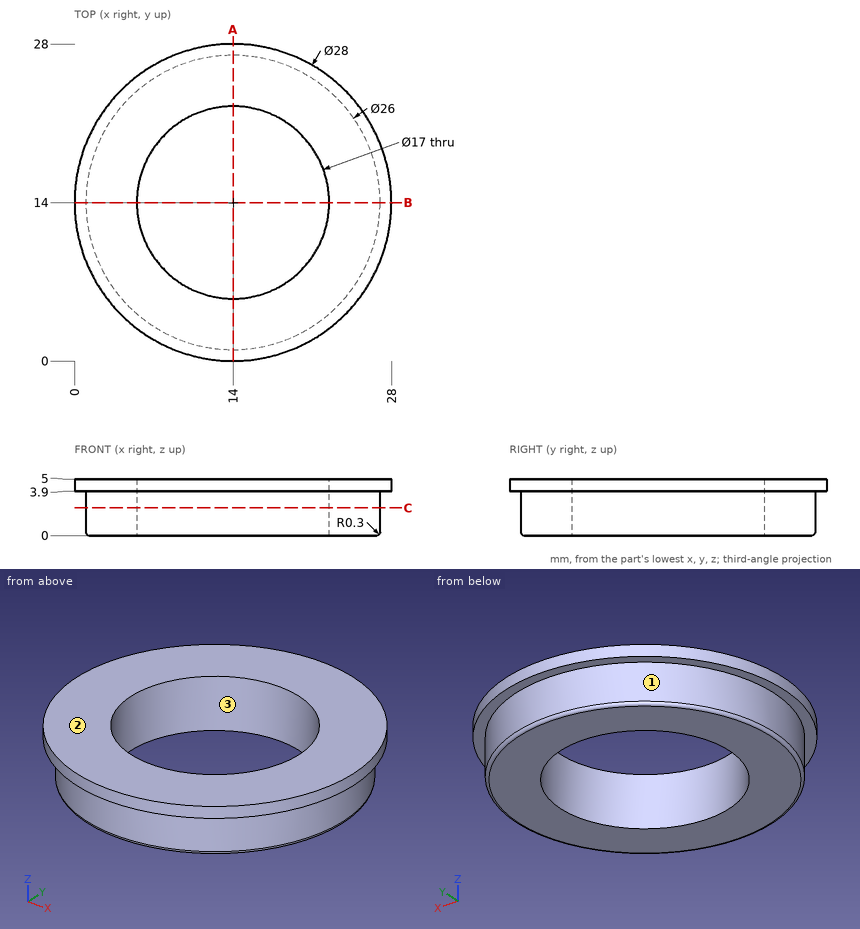
Study the drawing (mm; zero at the part's minimum x, y, z) and answer. Give positions to 0.01 mm unless a question says otherwise; leave off trailing zeros. Loops run counter-clockwise (first coordinate to the right, second up) from the corner with the lowest first, then second, coordinate; pieces in that order, holes last. Notation, with made-up numbers: (15, 30) - (51, 30) arc R26 ccw to (51, 49) - close; hole circle Ø8 at (66.25, -5). An arc over 180 degrees is marked (long way). Answer in a Markdown table with one row per item. Add a question column.
Q1. The part is cut by section A-A (x = 14). Determine the outline of the cut face in (y, z), and give its area (3 significant figures).
Q2. Determine the mould class of the marked faces 1, 2 and 3 for opening direction X: released by +X, released by -X, zero draft, split by the parting line, or undercut.
Q3. The part is cut by section C-C (z = 2.45). Determine the outline of the cut face in (x, y).
Q4. Each of these flat-tipped pins is pushed along its axis until it touches: P1, Ø2, axis at y = 4.5, z = 2, coming from the +X side; P2, Ø2, axis at y = 24, z = 4, coming from the -X side; P3, Ø1, axis at x = 4, z = 3.5, coming from the -Y side. Where does it stop, or does it pass through?
Q5. Consider line 1 along Y through (x, z) = (14, 3.75); line 2 along X through (y, z) = (10.5, 4); line 3 along Y through (x, z) = (15.75, 2.45). Determine where each line is inside the solid, lowest interval first.
Solution:
| question | item | result |
|---|---|---|
| 1 | outline | (0, 3.9) - (1, 3.9) - (1, 0.3) arc R0.3 ccw to (1.3, 0) - (5.5, 0) - (5.5, 5) - (0, 5) - close; (22.5, 0) - (26.7, 0) arc R0.3 ccw to (27, 0.3) - (27, 3.9) - (28, 3.9) - (28, 5) - (22.5, 5) - close |
| 1 | area | 47.2 mm² |
| 2 | face 1 | split by the parting line |
| 2 | face 2 | zero draft |
| 2 | face 3 | undercut |
| 3 | outline | circle Ø26 at (14, 14); hole circle Ø17 at (14, 14) |
| 4 | P1 | stops at x = 23.84 |
| 4 | P2 | stops at x = 3.28 |
| 4 | P3 | stops at y = 3.9 |
| 5 | line 1 | y = 1 to 5.5, 22.5 to 27 |
| 5 | line 2 | x = 0.44 to 6.25, 21.75 to 27.56 |
| 5 | line 3 | y = 1.12 to 5.68, 22.32 to 26.88 |
